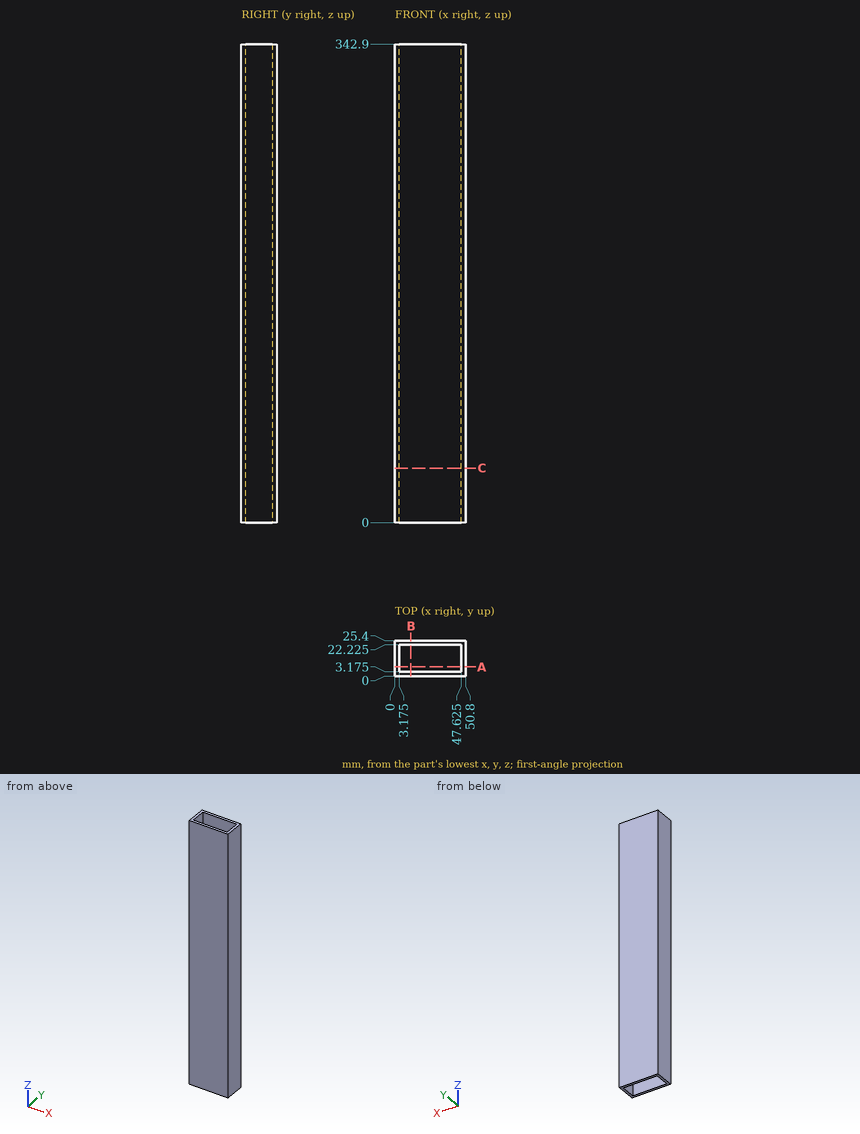
Could you check a few things on this drawing? It's one solid part, dimensions in mm from its lowest x, y, z. Round coordinates to 2 decimals unless told otherwise and drop trailing zeros. Order: outer loops, then holes, each group sorted by start corner. A loop starts at its lowest first (then second) coordinate and runs counter-clockwise, first axis right, second up.
(1) Please list where these lines run through material, in increasing order: line 1 along Y through (x, z) = (20, 208) (3 decimals); line 2 along X through (y, z) = (19, 184.5) (3 decimals).
Response values:
line 1: y = 0 to 3.175, 22.225 to 25.4
line 2: x = 0 to 3.175, 47.625 to 50.8
(2) Imagine slicing it at C-C (z = 39). Write out the boundary of the cut face in (x, y) (3 decimals).
Response values:
outline: (0, 0) - (50.8, 0) - (50.8, 25.4) - (0, 25.4) - close; hole (3.175, 3.175) - (47.625, 3.175) - (47.625, 22.225) - (3.175, 22.225) - close
(3) Imagine slicing it at B-B (x = 11.5). Write out the boundary of the cut face in (y, z) (3 decimals).
Response values:
outline: (0, 0) - (3.175, 0) - (3.175, 342.9) - (0, 342.9) - close; (22.225, 0) - (25.4, 0) - (25.4, 342.9) - (22.225, 342.9) - close
(4) Imagine slicing it at A-A (y = 6.5). Write out the boundary of the cut face in (x, z) (3 decimals), plus the area to 3 significant figures.
Response values:
outline: (0, 0) - (3.175, 0) - (3.175, 342.9) - (0, 342.9) - close; (47.625, 0) - (50.8, 0) - (50.8, 342.9) - (47.625, 342.9) - close
area: 2,180 mm2
